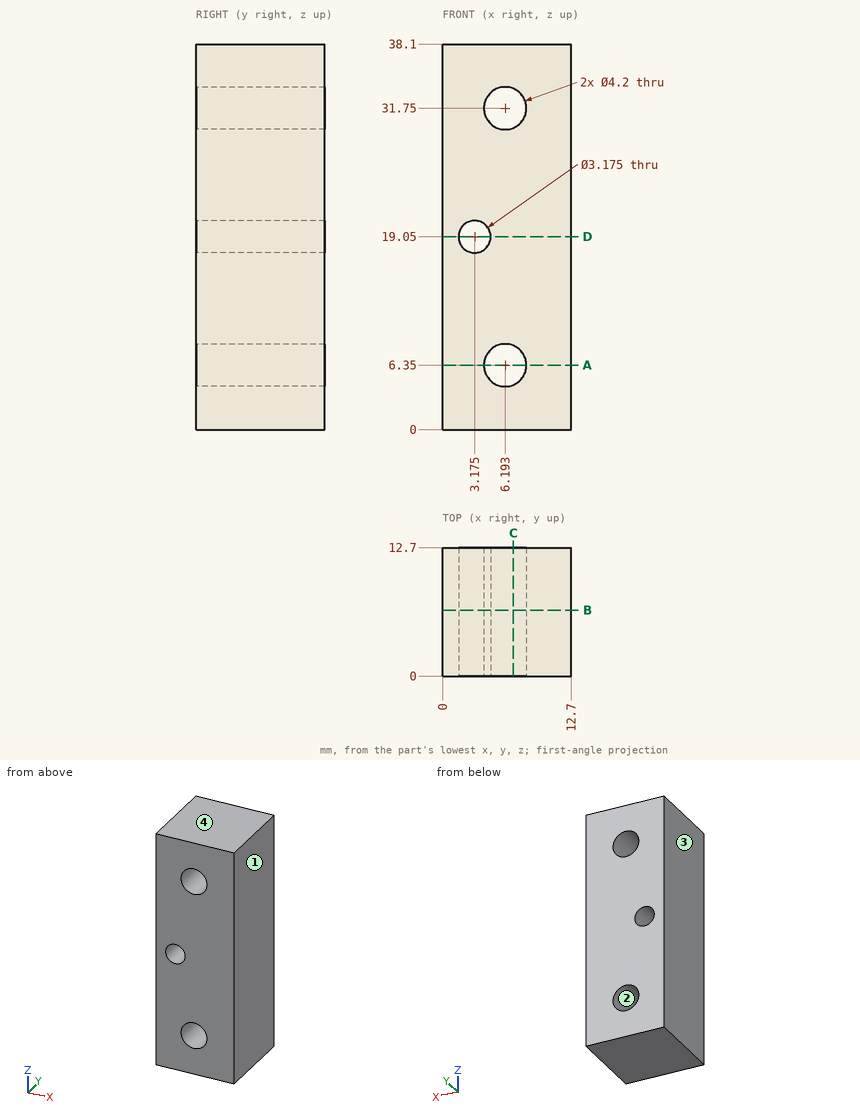
Could you check a few things on this drawing? It's one solid part, dimensions in mm from its lowest x, y, z. Give positions to 0.01 mm unless a question says otherwise; leave off trailing zeros. Order: outer loops, then holes, each group sorted by start corner. A loop starts at its lowest first (then second) coordinate and runs counter-clockwise, first axis right, second up. Notation, with made-up numbers: (35, 54) - (48, 54) arc R18 cw to (48, 68) - close; hole circle Ø6 at (-29.75, 44). An arc over 180 degrees is marked (long way). One line per item, written item: value. Start each with the question number.
1. For P1, Ø5.5, axis at x = 6.19, z = 31.75, coming from the -Y side, with a flat end and sliding along its axis, tell me the tip position at first contact or that it passes through.
2. Imagine slicing it at A-A on z = 6.35. List the corners of the cut face in (x, y) for me.
3. Imagine slicing it at C-C on x = 7. List the corners of the cut face in (y, z) for me, plus the area to 3 significant figures.
4. Imagine slicing it at D-D on z = 19.05. List the corners of the cut face in (x, y) for me, plus the area to 3 significant figures.
5. Imagine slicing it at B-B on y = 6.5. Give the number of separate pieces and of enclosed holes in the cut face, plus the area to 3 significant figures.
6. Thinking about a two-plate mould opening in X: for the marked faces 1, 2, 3 and 4, which applies, +X half, -X half, draft (parallel to the pull), parting line (faces both ways), or undercut?
7. If I drill on probe 1 along Z at (x, y) = (7.5, 1.75) (1 decimal); probe 2 along Z at (x, y) = (6.75, 0.5) (1 decimal); probe 3 along Z at (x, y) = (4.5, 4.75) (1 decimal), over which ranges is the centre line in solid material (lowest first)?
Values:
1. P1: y = 0
2. outline: (0, 0) - (4.09, 0) - (4.09, 12.7) - (0, 12.7) - close; (8.29, 0) - (12.7, 0) - (12.7, 12.7) - (8.29, 12.7) - close
3. outline: (0, 0) - (12.7, 0) - (12.7, 4.41) - (0, 4.41) - close; (0, 8.29) - (12.7, 8.29) - (12.7, 29.81) - (0, 29.81) - close; (0, 33.69) - (12.7, 33.69) - (12.7, 38.1) - (0, 38.1) - close
3. area: 385 mm²
4. outline: (0, 0) - (1.59, 0) - (1.59, 12.7) - (0, 12.7) - close; (4.76, 0) - (12.7, 0) - (12.7, 12.7) - (4.76, 12.7) - close
4. area: 121 mm²
5. separate pieces: 1
5. enclosed holes: 3
5. area: 448 mm²
6. face 1: +X half
6. face 2: undercut
6. face 3: -X half
6. face 4: draft
7. probe 1: 0 to 4.7, 8 to 30.1, 33.4 to 38.1
7. probe 2: 0 to 4.3, 8.4 to 29.7, 33.8 to 38.1
7. probe 3: 0 to 5.1, 7.6 to 18.2, 19.9 to 30.5, 33 to 38.1
